Source: three-view drawing plus pictorial views. Frame: mm from the lowest corner of the part. Give positions to 0.01 mm unless a question says otherwise; leave off trailing zeros. Order: outer loops, then holes, each group sorted by start corner. A loop starts at its lowest first (then second) coordinate and runs counter-clockwise, first axis right, second up. Notation, with made-up numbers: M 30.25,-16.75 L 46.25,-16.75 A16 ccw 46.25,7.25 Z; hole C -24,-9 d1. An arc over 180 degrees is marked long. Use CSV: the item, a comma, the result in double quotes. Start each with the question number.
1. Section query D-D, the plane x = 81.28. Return the cut outline in (y, z).
2. Section query B-B, the plane y = 52.07. Return the cut outline in (x, z), plus the area to 3 significant figures.
3. Line query: line 1 along Y through (x, z) = (81.28, 1.9); line 2 along Y through (x, z) = (3.81, 1.25). Output: solid intervals per line, ascending. Write a range as [from, to].
4. Section query A-A, the plane x = 3.81. Return the cut outline in (y, z).
5. Pin query (flat end, axial travel): P1, Ø2.5, axis at x = 81.28, y = 3.81, coming from the -Z side. Return the tip coordinate at first contact, or that it passes through.
6. Section query C-C, the plane y = 3.81. Return the cut outline in (x, z).
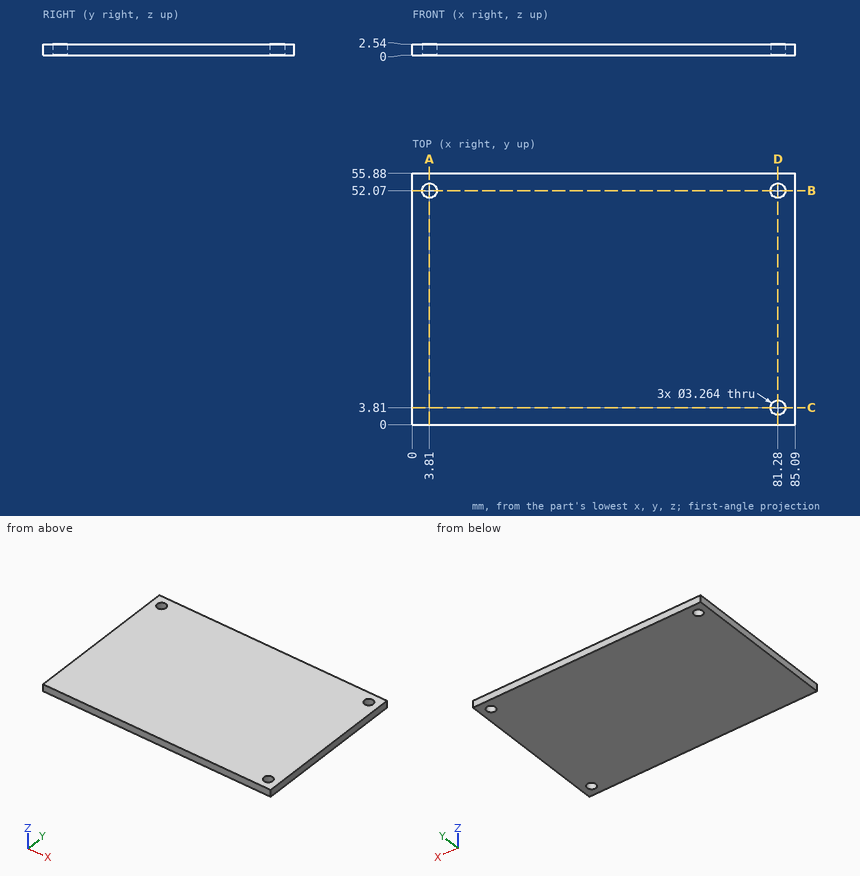
Result set:
1,outline,"M 0,0 L 2.18,0 L 2.18,2.54 L 0,2.54 Z; M 5.44,0 L 50.44,0 L 50.44,2.54 L 5.44,2.54 Z; M 53.7,0 L 55.88,0 L 55.88,2.54 L 53.7,2.54 Z"
2,outline,"M 0,0 L 2.18,0 L 2.18,2.54 L 0,2.54 Z; M 5.44,0 L 79.65,0 L 79.65,2.54 L 5.44,2.54 Z; M 82.91,0 L 85.09,0 L 85.09,2.54 L 82.91,2.54 Z"
2,area,"200 mm2"
3,line 1,"[0, 2.18], [5.44, 50.44], [53.7, 55.88]"
3,line 2,"[0, 50.44], [53.7, 55.88]"
4,outline,"M 0,0 L 50.44,0 L 50.44,2.54 L 0,2.54 Z; M 53.7,0 L 55.88,0 L 55.88,2.54 L 53.7,2.54 Z"
5,P1,"through"
6,outline,"M 0,0 L 79.65,0 L 79.65,2.54 L 0,2.54 Z; M 82.91,0 L 85.09,0 L 85.09,2.54 L 82.91,2.54 Z"
